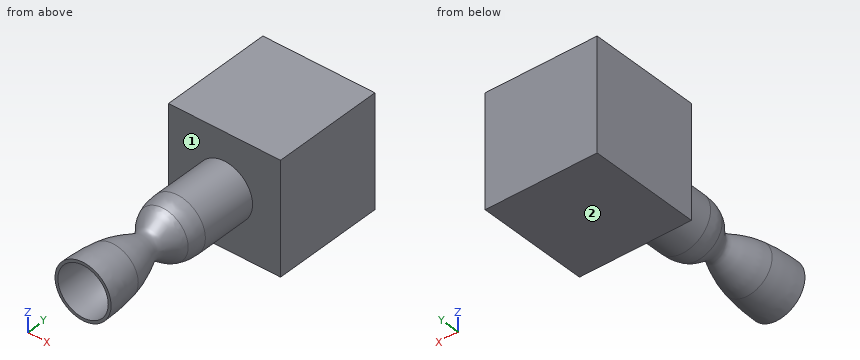
```python
from build123d import *

# Parameters (mm, degrees)
REVOLVE1_OUTLINE_W   = 5
REVOLVE1_OUTLINE_H   = 100
REVOLVE1_OUTLINE_W_2 = 45
SKETCH2_W            = 200
SKETCH2_H            = 200
BOSS_EXTRUDE1_DEPTH  = 200


# Read off the part's stored shape, not the designer's step: Revolve1
with BuildPart() as part:
    # Revolve1 outline → Revolve1 (revolve)
    with BuildSketch(Plane(origin=(50, 0, 0), x_dir=(1, 0, 0), z_dir=(0, 0, 1))):
        with Locations((47.5, 50)):
            Rectangle(REVOLVE1_OUTLINE_W, REVOLVE1_OUTLINE_H)
        with BuildLine():
            add(Edge.make_bspline(
                [(50, 0), (50, -8.082762567), (49.349957781, -15.002219913), (48.209745328, -20.96390459), (46.719575094, -26.132708235), (45, -30.644804173)],
                knots=[0, 0, 0, 0, 0, 0, 0.122970463, 0.122970463, 0.122970463, 0.122970463, 0.122970463, 0.122970463], degree=5))
            Line((50, 0), (45, 0))
            Line((45, 0), (45, -30.644804173))
        make_face()
        with Locations((22.5, 50)):
            Rectangle(REVOLVE1_OUTLINE_W_2, REVOLVE1_OUTLINE_H)
        with BuildLine():
            add(Edge.make_bspline(
                [(45, -30.644804173), (34.455506857, -58.313130409), (15.284968329, -61.288036888), (15.284968329, -70.967793904), (34.455506857, -78.145887533), (45, -136.380827106)],
                knots=[0.122970463, 0.122970463, 0.122970463, 0.122970463, 0.122970463, 0.122970463, 0.877029537, 0.877029537, 0.877029537, 0.877029537, 0.877029537, 0.877029537], degree=5))
            Line((45, -30.644804173), (45, 0))
            add(Edge.make_bspline(
                [(45, 0), (45, -0.805913513), (44.983206143, -2.440345101), (44.885909174, -5.527357683), (44.651249209, -9.180617017), (44.208693768, -13.22104238), (43.429179035, -18.197149025), (42.145056936, -23.699932493), (40.238749724, -29.339291486), (38.077480396, -34.180232479), (34.979043101, -39.765346635), (30.901795474, -45.44053167), (26.211141954, -50.99117289), (22.123818579, -55.99940601), (19.504937862, -60.49603289), (18.327366237, -64.615511375), (18.036096382, -67.865198675), (18.325954828, -71.151011846), (19.354041911, -75.549666709), (21.595505158, -81.301527469), (25.440968359, -89.686697726), (29.365247929, -98.822414083), (32.703100041, -108.024070812), (35.228496377, -116.046022636), (37.689368772, -125.375404851), (39.98622015, -136.217854158), (41.670948279, -146.701049549), (42.819586689, -156.079119992), (43.564957316, -163.641363627), (44.177194916, -171.766381725), (44.561675987, -179.035635061), (44.784641201, -185.169118612), (44.907191495, -189.931856825), (44.970095656, -194.044527702), (44.995668899, -197.414073857), (45, -199.141583294), (45, -200)],
                knots=[0, 0, 0, 0, 0.0078125, 0.015625, 0.03125, 0.046875, 0.0625, 0.09375, 0.125, 0.15625, 0.1875, 0.25, 0.3125, 0.375, 0.4375, 0.46875, 0.5, 0.53125, 0.5625, 0.625, 0.6875, 0.75, 0.78125, 0.8125, 0.84375, 0.875, 0.90625, 0.921875, 0.9375, 0.953125, 0.96875, 0.9765625, 0.984375, 0.9921875, 0.99609375, 1, 1, 1, 1], degree=3))
            Line((45, -200), (45, -136.380827106))
        make_face()
        with BuildLine():
            Line((45, -200), (50, -200))
            add(Edge.make_bspline(
                [(45, -136.380827106), (46.719575094, -145.877665912), (48.209745328, -156.732333022), (49.349957781, -169.177110028), (50, -183.488669983), (50, -200)],
                knots=[0.877029537, 0.877029537, 0.877029537, 0.877029537, 0.877029537, 0.877029537, 1, 1, 1, 1, 1, 1], degree=5))
            Line((45, -136.380827106), (45, -200))
        make_face()
    revolve(axis=Axis((50, 0, 0), (0, 1, 0)))

    # Sketch2 → Boss-Extrude1 (add)
    with BuildSketch(Plane(origin=(0, 100, 0), x_dir=(1, 0, 0), z_dir=(0, 1, 0))):
        with Locations((50, 0)):
            Rectangle(SKETCH2_W, SKETCH2_H)
    extrude(amount=BOSS_EXTRUDE1_DEPTH)


solid = part.part
```
Verification items for the finished model (mm, model axes). Face numbers are marked on the shaded views. A direction names the side the tool comes from. Round coordinates to 2 decimals unless told otherwise and drop trailing zeros. Order: outer loops, then holes, each group sorted by start corner. A loop starts at its lowest first (then second) coordinate and runs counter-clockwise, first axis right, second up.
1) Depth check by flat-ended pin: pin 1 (1 mm diameter, centred on x = 51.5, y = -71, fed in from -Z); pin 2 (2 mm diameter, centred on y = 63, z = -42, fed in from +X); pin 3 (8 mm diameter, centred on x = 56, y = 60.5, fed in from -Z). Enter the tip coordinate at first touch or a pass-through.
Geometry says:
pin 1: stops at z = -23.52
pin 2: stops at x = 78.62
pin 3: stops at z = -49.96
2) Material ranges on line 1 (Y direction, x = 67.5, z = 18.5); line 2 (Y direction, x = 123, z = 12); line 3 (Y direction, x = 51, z = -21), recorded low to high.
Geometry says:
line 1: y = -89.85 to -77.36, -60.32 to -51.92, 0 to 300
line 2: y = 100 to 300
line 3: y = -79.72 to -58.01, 0 to 300
3) Cross-section at C-C, the plane y = 92.5. Record the cut outline in (x, z), plus the area to 3 significant figures.
Geometry says:
outline: circle Ø100 at (50, 0)
area: 7,850 mm2
4) Tool access check on the marked faces 1 and 2. Record the directions out of +Z, -Z, +X, -X, +Y, -Y that give a thin tool (end or side, any length) a straight path to the whole face; none if there is none.
Geometry says:
face 1: -Y
face 2: -Z, +X, -X, +Y, -Y
5) Cross-section at A-A, the plane z = -31. Give the number of separate pieces and of enclosed holes in the cut face, plus the area to 3 significant figures.
Geometry says:
separate pieces: 2
enclosed holes: 1
area: 50,600 mm2
6) Cross-section at B-B, the plane z = -70. Record the cut outline in (x, y).
Geometry says:
outline: (-50, 100) - (150, 100) - (150, 300) - (-50, 300) - close
